Design review of the part built by this model. Coordinates are the model's own, in mm. Face numbers are marked on the shaded views. Coordinates: 2 decimals unless noted, no trailing zeros. Answer in a Markdown table with one row per item.
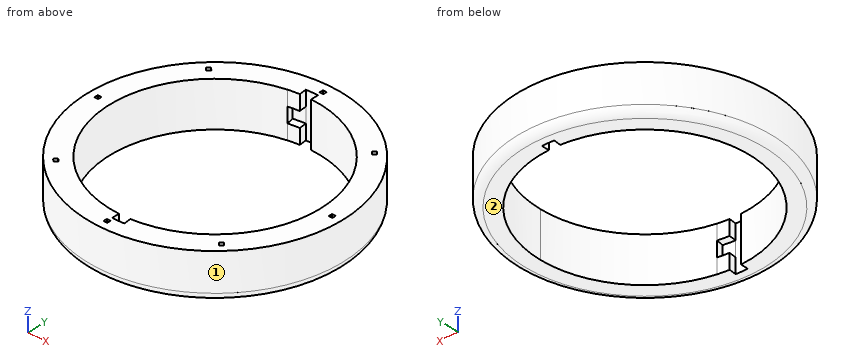
```python
from build123d import *

# Parameters (mm, degrees)
F0_R     = 85
F1_DEPTH = 30
F2_DEPTH = 10
F5_DEPTH = 10
F6_W     = 2.5
F6_H     = 2.5
F7_DEPTH = 20
F9_COUNT = 8
F11_R    = 5


with BuildPart() as f1:
    # F0 (on Top) → F1 (new body)
    with BuildSketch(Plane.XY):
        Circle(F0_R)
        with BuildLine():
            ThreePointArc((-7.8396347451, 74.5891421526), (-3.9251967182, 74.8972151066), (0, 75))
            ThreePointArc((0, 75), (53.033008589, 53.033008589), (75, 0))
            ThreePointArc((75, 0), (58.2859471093, -47.1990293287), (15.5933768113, -73.361070055))
            ThreePointArc((15.5933768113, -73.361070055), (11.732584878, -74.0766255446), (7.8396347451, -74.5891421526))
            ThreePointArc((7.8396347451, -74.5891421526), (3.9251967182, -74.8972151066), (0, -75))
            ThreePointArc((0, -75), (-74.5891421526, -7.8396347451), (-15.5933768113, 73.361070055))
            ThreePointArc((-15.5933768113, 73.361070055), (-11.732584878, 74.0766255446), (-7.8396347451, 74.5891421526))
        make_face(mode=Mode.SUBTRACT)
        with BuildLine():
            ThreePointArc((0, -70), (-69.6165326758, -7.3169924287), (-14.5538183572, 68.4703320514))
            Line((-14.5538183572, 68.4703320514), (-15.5933768113, 73.361070055))
            ThreePointArc((-15.5933768113, 73.361070055), (-74.5891421526, -7.8396347451), (0, -75))
            Line((0, -75), (0, -70))
        make_face()
        with BuildLine():
            ThreePointArc((0, 70), (49.4974746831, 49.4974746831), (70, 0))
            ThreePointArc((70, 0), (54.400217302, -44.0524273735), (14.5538183572, -68.4703320514))
            Line((14.5538183572, -68.4703320514), (15.5933768113, -73.361070055))
            ThreePointArc((15.5933768113, -73.361070055), (58.2859471093, -47.1990293287), (75, 0))
            ThreePointArc((75, 0), (53.033008589, 53.033008589), (0, 75))
            Line((0, 75), (0, 70))
        make_face()
    extrude(amount=F1_DEPTH)

    # F0 (on Top) → F2 (join)
    with BuildSketch(Plane.XY):
        with BuildLine():
            ThreePointArc((-14.5538183572, 68.4703320514), (-10.9504125528, 69.1381838417), (-7.3169924287, 69.6165326758))
            Line((-7.3169924287, 69.6165326758), (-7.8396347451, 74.5891421526))
            ThreePointArc((-7.8396347451, 74.5891421526), (-11.732584878, 74.0766255446), (-15.5933768113, 73.361070055))
            Line((-15.5933768113, 73.361070055), (-14.5538183572, 68.4703320514))
        make_face()
        with BuildLine():
            Line((15.5933768113, -73.361070055), (14.5538183572, -68.4703320514))
            ThreePointArc((14.5538183572, -68.4703320514), (10.9504125528, -69.1381838417), (7.3169924287, -69.6165326758))
            Line((7.3169924287, -69.6165326758), (7.8396347451, -74.5891421526))
            ThreePointArc((7.8396347451, -74.5891421526), (11.732584878, -74.0766255446), (15.5933768113, -73.361070055))
        make_face()
    extrude(amount=F2_DEPTH)

    # F4 (on offset) → F5 (join)
    with BuildSketch(Plane.XY.offset(20)):
        with BuildLine():
            Line((-7.3169924287, 69.6165326758), (-7.8396347451, 74.5891421526))
            ThreePointArc((-7.8396347451, 74.5891421526), (-11.732584878, 74.0766255446), (-15.5933768113, 73.361070055))
            Line((-15.5933768113, 73.361070055), (-14.5538183572, 68.4703320514))
            ThreePointArc((-14.5538183572, 68.4703320514), (-10.9504125528, 69.1381838417), (-7.3169924287, 69.6165326758))
        make_face()
        with BuildLine():
            ThreePointArc((7.8396347451, -74.5891421526), (11.732584878, -74.0766255446), (15.5933768113, -73.361070055))
            Line((15.5933768113, -73.361070055), (14.5538183572, -68.4703320514))
            ThreePointArc((14.5538183572, -68.4703320514), (10.9504125528, -69.1381838417), (7.3169924287, -69.6165326758))
            Line((7.3169924287, -69.6165326758), (7.8396347451, -74.5891421526))
        make_face()
    extrude(amount=F5_DEPTH)


with BuildPart() as f7:
    # F6 (on face) → F7 (new body, symmetric)
    with BuildSketch(Plane.XY.offset(30)):
        with Locations((0, 78.75)):
            Rectangle(F6_W, F6_H)
    extrude(amount=F7_DEPTH, both=True)


with BuildPart() as f9_1:
    # F9: instance of F7
    add(f7.part.rotate(Axis((0, 0, 11.2639116123), (0, 0, 1)), 1 * 360 / F9_COUNT))


with BuildPart() as f9_2:
    # F9: instance of F7
    add(f7.part.rotate(Axis((0, 0, 11.2639116123), (0, 0, 1)), 2 * 360 / F9_COUNT))


with BuildPart() as f9_3:
    # F9: instance of F7
    add(f7.part.rotate(Axis((0, 0, 11.2639116123), (0, 0, 1)), 3 * 360 / F9_COUNT))


with BuildPart() as f9_4:
    # F9: instance of F7
    add(f7.part.rotate(Axis((0, 0, 11.2639116123), (0, 0, 1)), 4 * 360 / F9_COUNT))


with BuildPart() as f9_5:
    # F9: instance of F7
    add(f7.part.rotate(Axis((0, 0, 11.2639116123), (0, 0, 1)), 5 * 360 / F9_COUNT))


with BuildPart() as f9_6:
    # F9: instance of F7
    add(f7.part.rotate(Axis((0, 0, 11.2639116123), (0, 0, 1)), 6 * 360 / F9_COUNT))


with BuildPart() as f9_7:
    # F9: instance of F7
    add(f7.part.rotate(Axis((0, 0, 11.2639116123), (0, 0, 1)), 7 * 360 / F9_COUNT))


with BuildPart() as f1_1:
    add(f1.part)

    # F10: cut F9_2, F9_1, F7, F9_7, F9_6, F9_5, F9_4, F9_3
    add(f9_2.part, mode=Mode.SUBTRACT)
    add(f9_1.part, mode=Mode.SUBTRACT)
    add(f7.part, mode=Mode.SUBTRACT)
    add(f9_7.part, mode=Mode.SUBTRACT)
    add(f9_6.part, mode=Mode.SUBTRACT)
    add(f9_5.part, mode=Mode.SUBTRACT)
    add(f9_4.part, mode=Mode.SUBTRACT)
    add(f9_3.part, mode=Mode.SUBTRACT)

    # F11
    f11_edges = [f1_1.edges().sort_by_distance(p)[0] for p in [
        (-85, 0, 0),
    ]]
    fillet(f11_edges, radius=F11_R)


solid = f1_1.part
```
(1) Draft analysis for pull direction Y (two halves, no side actions). For the marked faces 1 and 2, state which applies: pulls with the +Y half, pulls with the -Y half, needs draft (parallel to the pull), parting line crosses it, or undercut.
Evaluation:
| item | result |
|---|---|
| face 1 | parting line crosses it |
| face 2 | needs draft |
(2) To check wall thickness, follow probe 1 along X at (y, z) = (-44.5, 15); probe 2 along X at (y, z) = (39.5, 17); probe 3 along Y at (x, z) = (-56.5, 19.25). State the ranges of each line that lie inside material, in increasing order.
Evaluation:
| item | result |
|---|---|
| probe 1 | x = -72.42 to -54.03, 54.03 to 72.42 |
| probe 2 | x = -75.26 to -57.79, 57.79 to 75.26 |
| probe 3 | y = -63.5 to -56.64, -54.73 to -41.32, 41.32 to 54.73, 56.64 to 63.5 |
(3) For pin 1 (1.8 mm diameter, centred on x = 12.5, y = -70.5, fed in from -Z); pin 2 (1.5 mm diameter, centred on y = 31, z = 20.5, fed in from -X); pin 3 (0.8 mm diameter, centred on x = 78, z = 17.5, fed in from +Y); pin 4 (2 mm diameter, centred on x = -79, z = 22, fed in from -Y), all flat-tipped, find the tip position at first contact; note any pin that passes through.
Evaluation:
| item | result |
|---|---|
| pin 1 | stops at z = 0 |
| pin 2 | stops at x = -79.44 |
| pin 3 | stops at y = 34.69 |
| pin 4 | stops at y = -33.78 |
(4) Take a section at A-A on z = 25.5. Count the separate pieces of the cut face and the enclosed holes in it, and give its area (3 significant figures).
Evaluation:
| item | result |
|---|---|
| separate pieces | 1 |
| enclosed holes | 9 |
| area | 7,180 mm² |
